Autodesk Inventor part; units mm, degrees
ref_plane "YZ Plane" through (0, 0, 0) normal (1, 0, 0) x (0, 1, 0)
ref_plane "XZ Plane" through (0, 0, 0) normal (0, 1, 0) x (-1, 0, 0)
ref_plane "XY Plane" through (0, 0, 0) normal (0, 0, 1) x (1, 0, 0)
sketch "Sketch1" plane through (0, 0, 0) normal (0, 0, 1) x (1, 0, 0)
  circle A0 centre (0, 0) radius 26.5
  dimension "d0" = 53
extrude "Extrusion1" add sketch "Sketch1" along normal blind 8
sketch "Sketch2" plane through (0, 0, 8) normal (0, 0, 1) x (1, 0, 0)
  circle A0 centre (0, 0) radius 26.5
  circle A1 centre (0, 0) radius 4.25
  dimension "d3" = 8.5
extrude "Extrusion2" cut sketch "Sketch2" against normal blind 8 contours A1
sketch "Sketch3" plane through (0, 0, 8) normal (0, 0, 1) x (1, 0, 0)
  circle A0 centre (0, 0) radius 4.25
  circle A1 centre (0, 0) radius 26.5
  circle A2 centre (0, 0) radius 11.25
  dimension "d6" = 22.5
extrude "Extrusion3" cut sketch "Sketch3" against normal blind 7 contours A2
chamfer "Chamfer1" distance 1 angle 45 1 edges at (-11.25, 0, 8)
chamfer "Chamfer2" distance 1 angle 45 1 edges at (-26.5, 0, 8)
properties part number "SpoolHandle-wheel1"
Design review of the part built by this model. Coordinates are the model's own, in mm. A direction names the side the tool comes from. Round coordinates to 2 decimals unless told otherwise and drop trailing zeros. Write each loop counter-clockwise with the first axis right and the second up, starting at its lowest first coordinate (ties: lowest second). Pieces come first, ordered by that corner, then holes. Notation, with made-up numbers: (-19, 63.25) -> (16, 63.25) arc R28 ccw to (16, 95.25) -> close; hole circle Ø9 at (-34, -36). An arc over 180 degrees is marked (long way). Write item = value, one per line. Start each with the question number.
1) Mouldability with a two-part tool opening along Y and no side actions: class faces 3 (the face through (14.246, -22.345, 3.451)), 4 (the face through (2.285, 3.584, 0.507)), 5 (the face through (11, 6, 8)) as +Y half, -Y half, draft (parallel to the pull), parting line (faces both ways), or undercut.
2) Clearance check with flat-ended pins moving along their axes: pin 1 (3 mm diameter, centred on y = 7, z = 6.5, fed in from -X); pin 2 (1.5 mm diameter, centred on x = -2, z = 2, fed in from -Y); pin 3 (3 mm diameter, centred on x = 1, z = 5.5, fed in from +Y); pin 4 (7.5 mm diameter, centred on x = 0, y = 0, fed in from -Z). State where each tip first meets the part, or that it passes through.
3) Take a section at C-C, the plane z = 5.75. State the section outline as (x, y) points, plus the area to 3 significant figures.
4) Take a section at A-A, the plane x = 0. State the section outline as (y, z) points.
5) Tool access review of faces 1 (the face through (5.19, -9.98, 4.04)), 2 (the face through (6, 0, 0)): name each direction out of +Z, -Z, +X, -X, +Y, -Y from which nothing blocks a thin tool from reaching the whole face with its end or side.
6) Wall thickness on probe 1 along Y at (x, z) = (0, 0.65); probe 2 along X at (y, z) = (0.5, 6); probe 3 along X at (y, z) = (1.5, 3.25): over which ranges is each line inside the solid? List them lowest first. Write a range as from..to.
Results list:
q1.face_3 = parting line
q1.face_4 = undercut
q1.face_5 = draft
q2.pin_1 = -25.92
q2.pin_2 = -26.47
q2.pin_3 = 26.5
q2.pin_4 = through
q3.outline = circle Ø53 at (0, 0); hole circle Ø22.5 at (0, 0)
q3.area = 1,810 mm²
q4.outline = (-26.5, 0) -> (-4.25, 0) -> (-4.25, 1) -> (-11.25, 1) -> (-11.25, 7) -> (-12.25, 8) -> (-25.5, 8) -> (-26.5, 7) -> close; (4.25, 0) -> (26.5, 0) -> (26.5, 7) -> (25.5, 8) -> (12.25, 8) -> (11.25, 7) -> (11.25, 1) -> (4.25, 1) -> close
q5.face_1 = +Z
q5.face_2 = -Z, +X, -X, +Y, -Y
q6.probe_1 = -26.5..-4.25, 4.25..26.5
q6.probe_2 = -26.5..-11.24, 11.24..26.5
q6.probe_3 = -26.46..-11.15, 11.15..26.46
